Can you work these out from the model? Positions are in its coordinate system, mm. A direction names the side the tool comes from. Round coordinates to 2 decimals unless told otherwise and drop trailing zeros. Loops run counter-clockwise (first coordinate to the right, second up) from the corner with the lowest first, then second, coordinate; pieces in that order, holes last.
(1) If I drill on line 1 along Z through (x, y) = (20, -24); line 2 along Y through (x, z) = (16, 27.5); line 3 along Z through (x, y) = (15, -9), over which ranges is the centre line in solid material (lowest first)?
(2) I want a section at D-D on z = 22.5. Write out the boundary of the cut face in (x, y).
(3) Which directions (+Z, -Z, +X, -X, +Y, -Y) give clear straight access to the entire face, cutting with the end or side of a thin tool? Please do faces 1 (the face through (13, -25.4, 10)), 2 (the face through (15, -19, 19.05)).
(4) I want a section at B-B on z = 16.5. Write out the boundary of the cut face in (x, y), plus the area to 3 significant figures.
(5) I want a section at C-C on x = 19.5. Write out the boundary of the cut face in (y, z).
(6) I want a section at A-A on y = -11.5. Write out the boundary of the cut face in (x, z).
(7) Will these pins go through, and if not, where does the flat tip stop? pin 1 Ø10 at (x, y) = (29, -20) entering from -Z; pin 2 Ø4 at (y, z) = (-15, 29) entering from +X; pin 3 Ø6 at (x, z) = (7, 23.5) entering from -Y; pin 4 Ø6.5 at (x, y) = (23, -19) entering from +Z.
from build123d import *

# Parameters (mm, degrees)
F1_DEPTH = 25.4
F3_DEPTH = 38.100021
F5_DEPTH = 25.401
F7_DEPTH = 19.051


with BuildPart() as f1:
    # F0 (on Front) → F1 (new body)
    with BuildSketch(Plane.XZ):
        Polygon((38.099021, 38.1), (0, 38.373113), (0, 0), (38.099021, 0), align=None)
    extrude(amount=F1_DEPTH)

    # F2 (on Right) → F3 (cut, through all)
    with BuildSketch(Plane.YZ):
        Polygon((-12.7, 19.05), (-12.7, 38.488368), (-25.474755, 38.488368), (-25.453678, 19.05), align=None)
    extrude(amount=F3_DEPTH, mode=Mode.SUBTRACT)

    # F4 (on Front) → F5 (cut, through all)
    with BuildSketch(Plane.XZ):
        Polygon((38.132016, 38.228069), (25.06916, 38.420167), (38.132016, 19.594286), align=None)
    extrude(amount=F5_DEPTH, mode=Mode.SUBTRACT)

    # F6 (on face) → F7 (cut, through all)
    with BuildSketch(Plane.XY.offset(19.05)):
        Polygon((38.099021, -25.4), (38.099021, -12.7), (25.399021, -25.4), align=None)
    extrude(amount=-F7_DEPTH, mode=Mode.SUBTRACT)


solid = f1.part
Filled sheet:
1. line 1: z = 0 to 19.05
1. line 2: y = -12.7 to 0
1. line 3: z = 0 to 38.27
2. outline: (0, -12.7) - (36.12, -12.7) - (36.12, 0) - (0, 0) - close
3. face 1: +Z, -Z, +X, -X, -Y
3. face 2: +Z, +X, -X, -Y
4. outline: (0, -25.4) - (25.4, -25.4) - (38.1, -12.7) - (38.1, 0) - (0, 0) - close
4. area: 887 mm2
5. outline: (-25.4, 0) - (0, 0) - (0, 38.23) - (-12.7, 38.23) - (-12.7, 19.05) - (-25.4, 19.05) - close
6. outline: (0, 0) - (38.1, 0) - (38.1, 19.64) - (25.23, 38.19) - (0, 38.37) - close
7. pin 1: stops at z = 0
7. pin 2: passes through
7. pin 3: stops at y = -12.7
7. pin 4: stops at z = 19.05
